Can you work these out from the drawing? Everything is in mm from the part's minimum corner. A direction names the side the tool comes from. Coordinates: 2 decimals unless noted, no trailing zeros. Write each loop counter-clockwise with the first axis right and the second up, starting at its lowest first coordinate (ties: lowest second). Pieces come first, ordered by that corner, then holes.
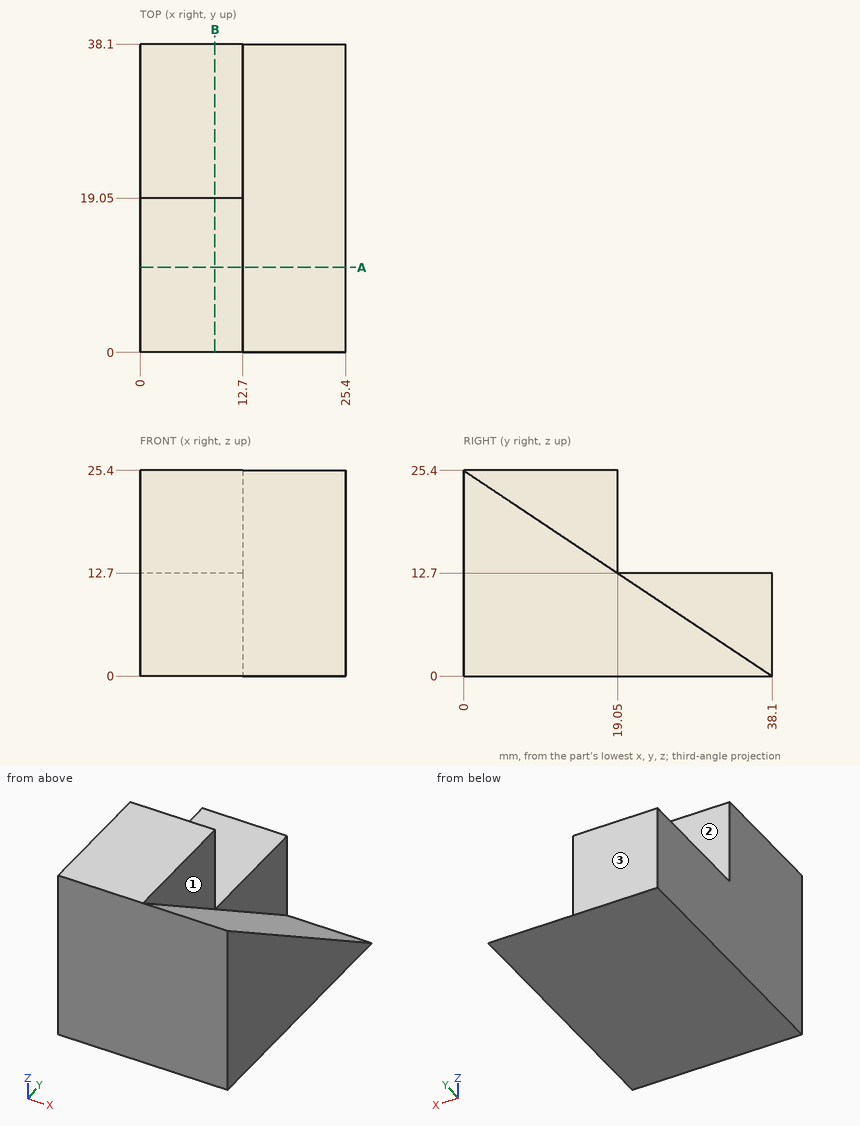
1. If I drill on line 1 (X direction, y = 33, z = 11); line 2 (Y direction, x = 7.5, z = 21.5), over which ranges is the centre line in solid material (lowest first)?
2. I want a section at B-B (x = 9.25). List the corners of the cut face in (y, z) for me.
3. For pin 1 Ø10 at (y, z) = (12, 21.5) entering from +X; pin 2 Ø1.5 at (x, z) = (20, 19) entering from +Y (3 decimals); pin 3 Ø4 at (x, y) = (5.5, 29) entering from +Z; pin 4 Ø1 at (x, y) = (20, 12) entering from +Z, each with a flat end and sliding along its axis, tell me the tip position at first contact or that it passes through.
4. On a 3-axis mill with a long thin cutter (end or side, diameter ignored), from which of +Z, -Z, +X, -X, +Y, -Y can I reach the whole of each face in a straight line? I mean the marked faces 1, 2 and 3. Say none if no direction works.
5. I want a section at A-A (y = 10.5). List the corners of the cut face in (x, z) for me, then the cut area to 3 significant figures.
Response values:
1. line 1: x = 0 to 12.7
1. line 2: y = 0 to 19.05
2. outline: (0, 0) - (38.1, 0) - (38.1, 12.7) - (19.05, 12.7) - (19.05, 25.4) - (0, 25.4) - close
3. pin 1: stops at x = 25.4
3. pin 2: stops at y = 10.725
3. pin 3: stops at z = 12.7
3. pin 4: stops at z = 17.73
4. face 1: +Z, +X, +Y
4. face 2: +Z, +X, -X, +Y
4. face 3: +Z, -Z, +X, -X, +Y
5. outline: (0, 0) - (25.4, 0) - (25.4, 18.4) - (12.7, 18.4) - (12.7, 25.4) - (0, 25.4) - close
5. area: 556 mm2
